```python
from build123d import *

# Parameters (mm, degrees)
F0_R     = 150
F1_DEPTH = 6
F2_W     = 6
F2_H     = 20
F3_DEPTH = 6.001


with BuildPart() as f1:
    # F0 (on Top) → F1 (new body)
    with BuildSketch(Plane.XY):
        Circle(F0_R)
    extrude(amount=F1_DEPTH)

    # F2 (on face) → F3 (cut, through all)
    with BuildSketch(Plane.XY.offset(6)):
        with Locations((-11, -125)):
            Rectangle(F2_W, F2_H)
        with Locations((11, -125)):
            Rectangle(F2_W, F2_H)
        Polygon((103.592921, 50.571797), (106.592921, 45.375644), (123.91343, 55.375644), (120.91343, 60.571797), align=None)
        Polygon((92.592921, 69.624356), (95.592921, 64.428203), (112.91343, 74.428203), (109.91343, 79.624356), align=None)
        Polygon((-95.592921, 64.428203), (-92.592921, 69.624356), (-109.91343, 79.624356), (-112.91343, 74.428203), align=None)
        Polygon((-106.592921, 45.375644), (-103.592921, 50.571797), (-120.91343, 60.571797), (-123.91343, 55.375644), align=None)
    extrude(amount=-F3_DEPTH, mode=Mode.SUBTRACT)


solid = f1.part
```
Could you check a few things on this model? Use its own coordinates, in mm. A direction names the side the tool comes from. Give positions to 0.01 mm unless a question says otherwise; leave off trailing zeros. Write each loop counter-clockwise with the first axis right and the second up, starting at its lowest first coordinate (ties: lowest second). Pieces come first, ordered by that corner, then holes. Notation, with made-up numbers: (12, 30) - (54, 30) arc R8 ccw to (54, 44) - close; hole circle Ø4 at (52, -29). An arc over 180 degrees is marked (long way). One line per item, written item: value. Start each with the question number.
Item 1: Which directions (+Z, -Z, +X, -X, +Y, -Y) give clear straight access to the entire face, cutting with the end or side of a thin tool? Please do faces 4 (the face through (-2, 2, 6)), 5 (the face through (104.132, 69.358, 3.042)).
Item 2: If we mould it in two halves opening along Y, with no side actions, what happens to faces 1 (the face through (112.37, 55.64, 3.04)), 2 (the face through (-19.527, 148.724, 2.958)), 3 (the face through (-2, 2, 0))? For each: +Y half, -Y half, draft (parallel to the pull), parting line (faces both ways), or undercut.
Item 3: Imagine slicing it at B-B, the plane x = -51. List the corners of the cut face in (y, z) for me, and give its area (3 significant figures).
Item 4: Please list where these lines run through material, in increasing order: line 1 (Y direction, x = 110.5, z = 2.25); line 2 (X direction, y = 102, z = 2.75); line 3 (Y direction, x = 118, z = 2.25). Write a range as from..to.
Item 5: I'm going to push flat-ended pins straight in: pin 1 (3 mm diameter, centred on y = -127, z = 3.5, fed in from -X); pin 2 (1.8 mm diameter, centred on x = 10.5, z = 4, fed in from -Y); pin 3 (1.5 mm diameter, centred on y = 66, z = 2, fed in from -X); pin 4 (2 mm diameter, centred on x = -3, y = -26.5, fed in from -Z). Where does each tip first touch, or does it pass through?
Item 6: Imagine slicing it at A-A, the plane y = 38.5. List the corners of the cut face in (x, z) for me (3 decimals), and give its area (3 significant figures).
Geometry says:
1. face 4: +Z, +X, -X, +Y, -Y
1. face 5: +Z, -Z
2. face 1: undercut
2. face 2: parting line
2. face 3: draft
3. outline: (-141.06, 0) - (141.06, 0) - (141.06, 6) - (-141.06, 6) - close
3. area: 1,690 mm^2
4. line 1: -101.44..47.63, 54.56..73.03, 78.61..101.44
4. line 2: -109.98..109.98
4. line 3: -92.61..51.96, 58.89..92.61
5. pin 1: x = -82.16
5. pin 2: y = -149.69
5. pin 3: x = -135.06
5. pin 4: z = 0
6. outline: (-144.975, 0) - (144.975, 0) - (144.975, 6) - (-144.975, 6) - close
6. area: 1,740 mm^2
